Read the model definition and answer for the solid it produces. Units are mm, in the model's axes. A direction names the side the tool comes from. Coordinates: 2 decimals unless noted, no trailing zeros. Loops run counter-clockwise (first coordinate to the right, second up) from the corner with the lowest first, then second, coordinate; pieces in that order, holes last.
Q1. Section A-A (x = 0) is taken. Give the vertices of the cut face in (y, z), then the cut area to 3 significant figures.
Q2. Section D-D (z = 26) is taken. Give the vertices of the cut face in (x, y), then the cut area to 3 significant figures.
Q3. Straight lines are drawn through the part: line 1 (Y direction, x = 17, z = 7); line 2 (Y direction, x = 23.75, z = 3.5). For each, find the intervals that lie inside material, in ascending order.
Q4. Section B-B (y = 0) is taken. Give the vertices of the cut face in (x, z), then the cut area to 3 significant figures.
Q5. Flat-ended cylindrical pins translate along their axes: P1, Ø11, axis at x = 0, y = 0, coming from the -Z side; P2, Ø1.5, axis at x = 15, y = 12, coming from the +Z side; P3, Ø12.5, axis at x = 4.5, y = -13, coming from the +Z side. Find the tip coordinate at first contact, or state that the pin passes through.
Q6. Section C-C (z = 71.5) is taken. Give the vertices of the cut face in (x, y), then the cut area to 3 significant figures.
Q7. The mould has two halves that part along Y. Classify faces 1 (the face through (15.63, -16.13, 5.98)), 2 (the face through (29, 0, 27)), 3 (the face through (0, 29, 39)): pulls with the +Y half, pulls with the -Y half, needs draft (parallel to the pull), parting line crosses it, or undercut.
Q8. Which of the six approach directions +Z, -Z, +X, -X, +Y, -Y give full straight-line access (tool end or side, diameter ignored) to faces 4 (the face through (-3.35, -0.44, 12.01)), 5 (the face through (0, -16, 45.066)), 6 (the face through (0, -29, 22))?
Autodesk Inventor part; units mm, degrees
ref_plane "YZ Plane" through (0, 0, 0) normal (1, 0, 0) x (0, 1, 0)
ref_plane "XZ Plane" through (0, 0, 0) normal (0, 1, 0) x (-1, 0, 0)
ref_plane "XY Plane" through (0, 0, 0) normal (0, 0, 1) x (1, 0, 0)
sketch "Sketch1" plane through (0, 0, 0) normal (0, 0, 1) x (1, 0, 0)
  line L0 (29, -29) -> (-29, -29)
  line L1 (-29, -29) -> (-29, 29)
  line L2 (-29, 29) -> (29, 29)
  line L3 (29, 29) -> (29, -29)
  line L4 (29, -29) -> (-29, 29) construction
  line L5 (-29, -29) -> (29, 29) construction
  point P0 (0, 0)
  point P1 (0, 0)
  dimension "d0" = 58
  dimension "d1" = 58
extrude "Extrusion1" add sketch "Sketch1" along normal blind 55.066
sketch "Sketch2" plane through (0, 0, 55.066) normal (0, 0, 1) x (1, 0, 0)
  line L0 (-29, 29) -> (-29, -29)
  line L1 (29, -29) -> (29, 29)
  line L2 (-29, -4) -> (29, -4)
  line L3 (29, -4) -> (29, -29)
  line L4 (29, -29) -> (-29, -29)
  line L5 (-29, -29) -> (-29, -4)
  point P0 (0, 0)
extrude "Extrusion2" cut sketch "Sketch2" against normal blind 10
hole "Hole1" at (0, 0, 0) direction (0, 0, 1) diameter 6.5 end through all
sketch "Sketch3" plane through (-29, 29, 0) normal (0, 1, 0) x (1, 0, 0)
  line L0 (0, 0) -> (58, 0)
  line L1 (0, 0) -> (0, -55.066)
  line L2 (58, -55.066) -> (0, -55.066)
  line L3 (58, 0) -> (58, -55.066)
  arc A0 (3.5064, -78.162) -> (54.3437, -78.162) centre (28.925, -94.0017) ccw
  line L4 (58, -55.066) -> (58, -45.066)
  line L5 (58, -55.066) -> (58.8673, -93.3229)
  line L6 (0, -45.066) -> (0, -55.066)
  line L7 (0, -55.066) -> (-1.0173, -94.6805)
  line L8 (58.5236, -78.162) -> (-0.5931, -78.162)
  arc A1 (54.3437, -78.162) -> (3.5064, -78.162) centre (28.925, -94.0017) ccw
  point P0 (29, 0)
  dimension "d13" = 59.9
extrude "Extrusion3" add sketch "Sketch3" against normal blind 5 contours L2 L5 L8 A1 L7
hole "Hole2" at (0, 0, 0) direction (0, 0, 1) diameter 6.756 depth 13 tip angle 118 counterbore diameter 11.113 counterbore depth 11
sketch "Sketch4" plane through (0, 0, 0) normal (0, 0, -1) x (-1, 0, 0)
  line L0 (-23.75, 23.75) -> (23.75, 23.75)
  line L1 (23.75, 23.75) -> (23.75, -23.75)
  line L2 (23.75, -23.75) -> (-23.75, -23.75)
  line L3 (-23.75, -23.75) -> (-23.75, 23.75)
  line L4 (-23.75, 23.75) -> (23.75, -23.75) construction
  line L5 (23.75, 23.75) -> (-23.75, -23.75) construction
  line L6 (-14.6492, 0) -> (14.3408, 0)
  point P0 (0, 0)
  point P1 (-17, -17)
  point P2 (17, -17)
  point P3 (-17, 17)
  point P4 (17, 17)
  dimension "d23" = 47.5
  dimension "d24" = 47.5
  dimension "d33" = 34
  dimension "d36" = 34
  dimension "d39" = 34
hole "Hole3" at (-23.75, -23.75, 0) at (23.75, -23.75, 0) at (-23.75, 23.75, 0) at (23.75, 23.75, 0) direction (0, 0, 1) diameter 2.459 depth 8.8 tip angle 118
hole "Hole4" at (17, -17, 0) at (17, 17, 0) at (-17, 17, 0) at (-17, -17, 0) direction (0, 0, 1) diameter 3.242 depth 11.8 tip angle 118
properties part number "Iris15-XT66P2M_H94mm(axis2base)"
Numbers:
1. outline: (-29, 0) - (-5.56, 0) - (-5.56, 11) - (-3.38, 11) - (-3.38, 13) - (-3.25, 13.08) - (-3.25, 55.07) - (-4, 55.07) - (-4, 45.07) - (-29, 45.07) - close; (3.25, 13.08) - (3.38, 13) - (3.38, 11) - (5.56, 11) - (5.56, 0) - (29, 0) - (29, 64.05) - (24, 64.05) - (24, 55.07) - (3.25, 55.07) - close
1. area: 2,580 mm2
2. outline: (-29, -29) - (29, -29) - (29, 29) - (-29, 29) - close; hole circle Ø6.5 at (0, 0)
2. area: 3,330 mm2
3. line 1: y = -29 to -18.62, -15.38 to 15.38, 18.62 to 29
3. line 2: y = -29 to -24.98, -22.52 to 22.52, 24.98 to 29
4. outline: (-29, 0) - (-5.56, 0) - (-5.56, 11) - (-3.38, 11) - (-3.38, 13) - (-3.25, 13.08) - (-3.25, 55.07) - (-29, 55.07) - close; (3.25, 13.08) - (3.38, 13) - (3.38, 11) - (5.56, 11) - (5.56, 0) - (29, 0) - (29, 55.07) - (3.25, 55.07) - close
4. area: 2,780 mm2
5. P1: stops at z = 11
5. P2: stops at z = 55.07
5. P3: stops at z = 45.07
6. outline: (-29.42, 24) - (-19.84, 24) - (-19.84, 29) - (-29.42, 29) - close; (19.69, 24) - (29.37, 24) - (29.37, 29) - (19.69, 29) - close
6. area: 96.3 mm2
7. face 1: undercut
7. face 2: needs draft
7. face 3: pulls with the +Y half
8. face 4: -Z
8. face 5: +Z, +X, -X, -Y
8. face 6: +Z, -Z, +X, -X, -Y
